Check sheet for the modelled part. Datum: model origin and axes. Units: mm. Face numbers are marked on the shaded views. Give positions to 0.01 mm unless a question says otherwise; leave off trailing zeros. Order: outer loops, then holes, each group sorted by start corner. A loop starts at its lowest first (then second) coordinate and runs counter-clockwise, first axis right, second up. Notation, with made-up numbers: (-16.75, 67) -> (34.25, 67) arc R21 ccw to (34.25, 94) -> close; hole circle Ø1 at (4.5, 54). An arc over 180 degrees is marked (long way). Answer in a Markdown table with one row per item. Add a question column.
(1) Thickness scan on L1, parallel to Y at x = 6, z = 12.25; L2, parallel to Y at x = 143, z = 4.75; L3, parallel to Y at x = 80, z = 1.75. Record the ranges inside material, lowest first. Write a range as [from, to].
(2) Release check for a two-part mould opening along X. For the marked faces 1 and 2 record: released by +X, released by -X, zero draft, split by the parting line, or undercut.
(3) Go/stop test with a flat-tipped pin: pin 1 (8.5 mm diameter, centred on x = 154, y = -6, fed in from -Z). Record where the tip stops, or that it passes through.
(4) Cross-section at A-A (x = 113). Record the cut outline in (y, z), then the cut area to 3 significant figures.
(5) Cross-section at C-C (x = 6). Record the cut outline in (y, z), then the cut area to 3 significant figures.
(6) Cross-section at D-D (y = -54.25). Record the cut outline in (x, z).
(7) Cross-section at B-B (z = 13). State how many separate pieces and enclosed holes the cut face has, then the cut area to 3 significant figures.
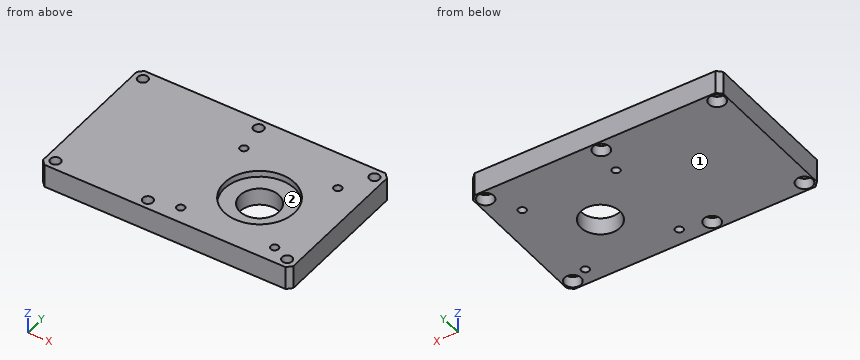
```python
from build123d import *

# Parameters (mm, degrees)
SKETCH_1_W             = 160
SKETCH_1_H             = 95
EXTRUDE_1_DEPTH        = 15
CHAMFER_1_SIZE         = 3
SKETCH_2_R             = 12.5
CUT_EXTRUDE_1_DEPTH    = 16
HOLE_WIZARD_M6_1_D     = 5
HOLE_WIZARD_M6_1_DEPTH = 20
HOLE_WIZARD_M6_1_TIP   = 1.502151548
SKETCH_6_R             = 5.25
CUT_EXTRUDE_2_DEPTH    = 7
SKETCH_7_R             = 3.25
CUT_EXTRUDE_3_DEPTH    = 9
SKETCH_8_R             = 22.5
CUT_EXTRUDE_4_DEPTH    = 4


with BuildPart() as part:
    # 草图1 → 凸台-拉伸1 (new body)
    with BuildSketch(Plane.XY):
        with Locations((80, -47.5)):
            Rectangle(SKETCH_1_W, SKETCH_1_H)
    extrude(amount=EXTRUDE_1_DEPTH)

    # 倒角1
    chamfer_1_edges = [part.edges().sort_by_distance(p)[0] for p in [
        (0, 0, 7.5),
        (160, 0, 7.5),
        (160, -95, 7.5),
        (0, -95, 7.5),
    ]]
    chamfer(chamfer_1_edges, length=CHAMFER_1_SIZE)

    # 草图2 → 切除-拉伸1 (cut, through all)
    with BuildSketch(Plane(origin=(0, 0, 0), x_dir=(-1, 0, 0), z_dir=(0, 0, -1))):
        with Locations((-113, -54.25)):
            Circle(SKETCH_2_R)
    extrude(amount=-CUT_EXTRUDE_1_DEPTH, mode=Mode.SUBTRACT)

    # M6 螺纹孔1
    with Locations(Plane(origin=(0, 0, 0), x_dir=(-1, 0, 0), z_dir=(0, 0, -1))):
        with Locations((-143, -24.5), (-83, -24.5), (-83, -84.5), (-143, -84.5)):
            Hole(HOLE_WIZARD_M6_1_D / 2, depth=HOLE_WIZARD_M6_1_DEPTH)
            with Locations((0, 0, -(HOLE_WIZARD_M6_1_DEPTH + HOLE_WIZARD_M6_1_TIP / 2))):  # 118° drill point
                Cone(0, HOLE_WIZARD_M6_1_D / 2, HOLE_WIZARD_M6_1_TIP, mode=Mode.SUBTRACT)

    # 草图6 → 切除-拉伸2 (cut)
    with BuildSketch(Plane(origin=(0, 0, 0), x_dir=(-1, 0, 0), z_dir=(0, 0, -1))):
        with Locations((-154, -6)):
            Circle(SKETCH_6_R)
        with Locations((-80, -6)):
            Circle(SKETCH_6_R)
        with Locations((-6, -6)):
            Circle(SKETCH_6_R)
        with Locations((-6, -89)):
            Circle(SKETCH_6_R)
        with Locations((-154, -89)):
            Circle(SKETCH_6_R)
        with Locations((-65, -89)):
            Circle(SKETCH_6_R)
    extrude(amount=-CUT_EXTRUDE_2_DEPTH, mode=Mode.SUBTRACT)

    # 草图7 → 切除-拉伸3 (cut, through all)
    with BuildSketch(Plane(origin=(0, 0, 7), x_dir=(-1, 0, 0), z_dir=(0, 0, -1))):
        with Locations((-154, -6)):
            Circle(SKETCH_7_R)
        with Locations((-80, -6)):
            Circle(SKETCH_7_R)
        with Locations((-6, -6)):
            Circle(SKETCH_7_R)
        with Locations((-6, -89)):
            Circle(SKETCH_7_R)
        with Locations((-154, -89)):
            Circle(SKETCH_7_R)
        with Locations((-65, -89)):
            Circle(SKETCH_7_R)
    extrude(amount=-CUT_EXTRUDE_3_DEPTH, mode=Mode.SUBTRACT)

    # 草图8 → 切除-拉伸4 (cut)
    with BuildSketch(Plane.XY.offset(15)):
        with Locations((113, -54.25)):
            Circle(SKETCH_8_R)
    extrude(amount=-CUT_EXTRUDE_4_DEPTH, mode=Mode.SUBTRACT)


solid = part.part
```
Answer below:
| question | item | result |
|---|---|---|
| 1 | L1 | y = [-95, -92.25], [-85.75, -9.25], [-2.75, 0] |
| 1 | L2 | y = [-95, -87], [-82, -27], [-22, 0] |
| 1 | L3 | y = [-95, -11.25], [-0.75, 0] |
| 2 | face 1 | zero draft |
| 2 | face 2 | undercut |
| 3 | pin 1 | stops at z = 7 |
| 4 | outline | (-95, 0) -> (-66.75, 0) -> (-66.75, 11) -> (-76.75, 11) -> (-76.75, 15) -> (-95, 15) -> close; (-41.75, 0) -> (0, 0) -> (0, 15) -> (-31.75, 15) -> (-31.75, 11) -> (-41.75, 11) -> close |
| 4 | area | 970 mm² |
| 5 | outline | (-95, 0) -> (-94.25, 0) -> (-94.25, 7) -> (-92.25, 7) -> (-92.25, 15) -> (-95, 15) -> close; (-85.75, 7) -> (-83.75, 7) -> (-83.75, 0) -> (-11.25, 0) -> (-11.25, 7) -> (-9.25, 7) -> (-9.25, 15) -> (-85.75, 15) -> close; (-2.75, 7) -> (-0.75, 7) -> (-0.75, 0) -> (0, 0) -> (0, 15) -> (-2.75, 15) -> close |
| 5 | area | 1,170 mm² |
| 6 | outline | (0, 0) -> (100.5, 0) -> (100.5, 11) -> (90.5, 11) -> (90.5, 15) -> (0, 15) -> close; (125.5, 0) -> (160, 0) -> (160, 15) -> (135.5, 15) -> (135.5, 11) -> (125.5, 11) -> close |
| 7 | separate pieces | 1 |
| 7 | enclosed holes | 11 |
| 7 | area | 13,300 mm² |
